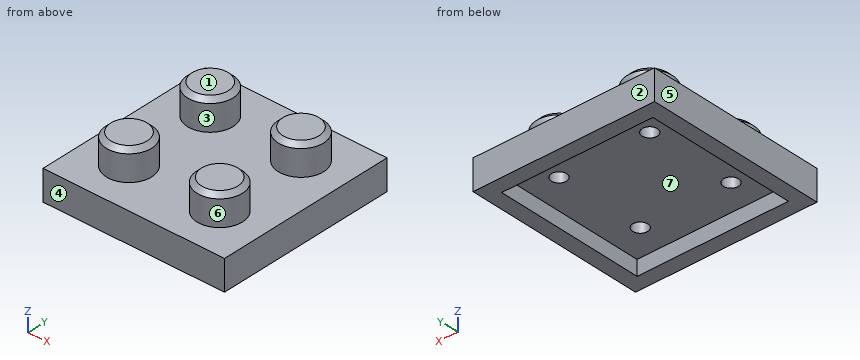
from build123d import *

# Parameters (mm, degrees)
F3_W     = 12
F3_H     = 12
F0_DEPTH = 2
F1_R     = 1.5
F4_DEPTH = 2
F5_SIZE  = 0.3
F2_T     = 1


# Not quite as in the source:
# - a shell that OpenCascade refuses in one call is made with other operations: the cavity is built on its own and cut out


with BuildPart() as f0:
    # F3 (on Top) → F0 (new body)
    with BuildSketch(Plane.XY):
        Rectangle(F3_W, F3_H)
    extrude(amount=-F0_DEPTH)

    # F1 (on Top) → F4 (join)
    with BuildSketch(Plane.XY):
        with Locations((3, 3)):
            Circle(F1_R)
        with Locations((-3, 3)):
            Circle(F1_R)
        with Locations((3, -3)):
            Circle(F1_R)
        with Locations((-3, -3)):
            Circle(F1_R)
    extrude(amount=F4_DEPTH)

    # F5
    f5_edges = [f0.edges().sort_by_distance(p)[0] for p in [
        (-4.5, 3, 2),
        (1.5, 3, 2),
        (-4.5, -3, 2),
        (1.5, -3, 2),
    ]]
    chamfer(f5_edges, length=F5_SIZE)

    # F2: shell of thickness 1, made by hand


with BuildPart() as f2_core1:
    # F2_t2: copy of F0
    add(f0.part)

    # the walls: a layer under each face that stays
    f2_faces = [f2_core1.faces().sort_by_distance(p)[0] for p in [
        (-4.5, -3, 0.85),
        (-4.35, -3, 1.85),
        (0, 0, 0),
        (-3, -3, 2),
        (0, 6, -1),
        (6, 0, -1),
        (-6, 0, -1),
        (0, -6, -1),
        (1.5, -3, 0.85),
        (-4.5, 3, 0.85),
        (1.5, 3, 0.85),
        (1.65, -3, 1.85),
        (-4.35, 3, 1.85),
        (1.65, 3, 1.85),
        (3, -3, 2),
        (-3, 3, 2),
        (3, 3, 2),
    ]]
    thicken(f2_faces, amount=-F2_T, mode=Mode.SUBTRACT)

    # F2_s3 → F2_t4 (revolve, cut)
    with BuildSketch(Plane.XZ.offset(3)):
        Polygon((-1.49, 0.01), (-2.5, 0), (-2.5, -1), (-1.5, -1), align=None)
    revolve(axis=Axis((-3, -3, 0), (0, 0, 1)), mode=Mode.SUBTRACT)

    # F2_s5 → F2_t6 (revolve, cut)
    with BuildSketch(Plane.XZ.offset(3)):
        Polygon((4.51, 0.01), (4.5, -1), (3.5, -1), (3.5, 0), align=None)
    revolve(axis=Axis((3, -3, 0), (0, 0, 1)), mode=Mode.SUBTRACT)

    # F2_s7 → F2_t8 (revolve, cut)
    with BuildSketch(Plane.XZ.offset(-3)):
        Polygon((-1.49, 0.01), (-1.5, -1), (-2.5, -1), (-2.5, 0), align=None)
    revolve(axis=Axis((-3, 3, 0), (0, 0, 1)), mode=Mode.SUBTRACT)

    # F2_s9 → F2_t10 (revolve, cut)
    with BuildSketch(Plane.XZ.offset(-3)):
        Polygon((4.51, 0.01), (4.5, -1), (3.5, -1), (3.5, 0), align=None)
    revolve(axis=Axis((3, 3, 0), (0, 0, 1)), mode=Mode.SUBTRACT)


with BuildPart() as f0_1:
    add(f0.part)

    # what is left inside the walls is the cavity
    f2_cavity = [f2_core1.part.solids().sort_by_distance(p)[0] for p in [
        (0, -1.666667, -1.99),
    ]]
    add(f2_cavity, mode=Mode.SUBTRACT)


solid = f0_1.part
Read the model definition and answer for the solid it produces. Units are mm, in the model's axes. Face numbers are marked on the shaded views. A direction names the side the tool comes from. Give positions to 0.01 mm unless a question says otherwise; leave off trailing zeros. Write each loop counter-clockwise with the first axis right and the second up, starting at its lowest first coordinate (ties: lowest second). Pieces come first, ordered by that corner, then holes. Notation, with made-up numbers: (62.5, 19) -> (92.5, 19) arc R20 cw to (92.5, 49) -> close; hole circle Ø6 at (40.5, 52). An arc over 180 degrees is marked (long way). Answer as a JSON object with one key per item and string values. Group by question number.
1) Consider L1, parallel to Y at x = -3, z = -0.2; L2, parallel to Y at x = -3, z = 0.5. Determine where each line is inside the solid, lowest interval first. Write a range as from..to.
2) Find section C-C (z = 1.4). Write down the section's boundary in (x, y).
3) Find section B-B (y = -1.25). Write down the section's boundary in (x, z), and give its area (3 significant figures).
4) A tool of negligible diameter and unlimited length cuts with its end or side. For the marked faces 5, 6 and 7, from which of +Z, -Z, +X, -X, +Y, -Y can it reach the whole face along a straight path? Write none if from no direction.
5) The mould has two halves that part along Y. Classify the marked faces 1, 2, 3 and 4: +Y half, -Y half, draft (parallel to the pull), parting line (faces both ways), or undercut.
6) Each of these flat-tipped pins is pushed along its axis until it touches: P1, Ø3, axis at x = 0, y = -1, coming from the -Z side; P2, Ø0.5, axis at x = -3, y = 3, coming from the -Z side; P3, Ø2, axis at x = -0.5, y = -4.5, coming from the -Z side. Where does it stop, or does it pass through?
7) Find section A-A (z = 0.6). Write down the section's boundary in (x, y), and give its area (3 significant figures).
8) Find section D-D (x = -3). Write down the section's boundary in (y, z), and give its area (3 significant figures).
Values follow:
{
 "1": {"L1": "y = -6..-3.5, -2.5..2.5, 3.5..6", "L2": "y = -4.5..-3.5, -2.5..-1.5, 1.5..2.5, 3.5..4.5"},
 "2": {"outline": "circle Ø3 at (-3, -3); circle Ø3 at (-3, 3); circle Ø3 at (3, -3); circle Ø3 at (3, 3)"},
 "3": {"outline": "(-6, -2) -> (-5, -2) -> (-5, -1) -> (5, -1) -> (5, -2) -> (6, -2) -> (6, 0) -> (-6, 0) -> close", "area": "14.0 mm2"},
 "4": {"face 5": "+Z, -Z, -X, +Y, -Y", "face 6": "+Z", "face 7": "-Z"},
 "5": {"face 1": "draft", "face 2": "+Y half", "face 3": "undercut", "face 4": "-Y half"},
 "6": {"P1": "stops at z = -1", "P2": "stops at z = 1", "P3": "stops at z = -2"},
 "7": {"outline": "circle Ø3 at (-3, -3); circle Ø3 at (-3, 3); circle Ø3 at (3, -3); circle Ø3 at (3, 3); hole circle Ø1 at (-3, -3); hole circle Ø1 at (-3, 3); hole circle Ø1 at (3, -3); hole circle Ø1 at (3, 3)", "area": "25.1 mm2"},
 "8": {"outline": "(-6, -2) -> (-5, -2) -> (-5, -1) -> (-3.5, -1) -> (-3.5, 1) -> (-2.5, 1) -> (-2.5, -1) -> (2.5, -1) -> (2.5, 1) -> (3.5, 1) -> (3.5, -1) -> (5, -1) -> (5, -2) -> (6, -2) -> (6, 0) -> (4.5, 0) -> (4.5, 1.7) -> (4.2, 2) -> (1.8, 2) -> (1.5, 1.7) -> (1.5, 0) -> (-1.5, 0) -> (-1.5, 1.7) -> (-1.8, 2) -> (-4.2, 2) -> (-4.5, 1.7) -> (-4.5, 0) -> (-6, 0) -> close", "area": "21.8 mm2"}
}
